Could you check a few things on this model? Use its own coordinates, in mm. A direction names the side the tool comes from. Give positions to 0.01 mm unless a question says otherwise; leave off trailing zeros. Order: outer loops, then holes, each group sorted by start corner. A loop starts at its lowest first (then second) coordinate and runs counter-clockwise, first axis right, second up. Notation, with made-up numbers: (29.25, -32) -> (34.25, -32) arc R10 ccw to (34.25, -21) -> close; hole circle Ø3 at (83.5, 9.5). An arc over 180 degrees is marked (long way). Answer as CSV lines item,"result". Start each with the question number.
(1) I need wall thicknesses on L1, parallel to X at y = 8.75, z = -36; L2, parallel to Z at x = -69, y = 4.5; L3, parallel to X at y = 8, z = 90.5. Which ranges of each line are inside material? Lowest first, please.
(2) I want a section at A-A (z = 49.5). Please give me the cut outline in (x, y).
(3) Will this pin go through, and if not, where does the flat tip stop? pin 1 Ø1 at (x, y) = (3.5, 7.5) entering from +Z.
(4) I want a section at B-B (y = 6.75). Give the number of separate pieces and of enclosed holes in the cut face, plus the area to 3 significant figures.
(5) On a 3-axis mill with a long thin cutter (end or side, diameter ignored), from which of +Z, -Z, +X, -X, +Y, -Y can I reach the whole of each face in a straight line? I mean faces 4 (the face through (-21.359, 6.056, -8.797)), 5 (the face through (-25.047, 6, 89)). Say none if no direction works.
(6) We'd pull the mould along Z, two halves only. Please class faces 1 (the face through (1, 1.6, 100)), 2 (the face through (1, 0, -1)), 3 (the face through (32, 6, 55.357)): released by +Z, released by -Z, zero draft, split by the parting line, or undercut.
```python
from build123d import *

# Parameters (mm, degrees)
EXTRUDE_1_DEPTH     = 10
CUT_EXTRUDE_1_DEPTH = 8
SKETCH_3_R          = 1.5875
CUT_EXTRUDE_2_DEPTH = 126.39936204


with BuildPart() as part:
    # Эскиз1 → Бобышка-Вытянуть1 (new body)
    with BuildSketch(Plane(origin=(0, 0, 0), x_dir=(1, 0, 0), z_dir=(0, 1, 0))):
        with BuildLine():
            Line((-72, 100), (72, 100))
            ThreePointArc((72, 100), (74.121320344, 99.121320344), (75, 97))
            Line((75, 97), (75, -97))
            ThreePointArc((75, -97), (74.121320344, -99.121320344), (72, -100))
            Line((72, -100), (-72, -100))
            ThreePointArc((-72, -100), (-74.121320344, -99.121320344), (-75, -97))
            Line((-75, -97), (-75, 97))
            ThreePointArc((-75, 97), (-74.121320344, 99.121320344), (-72, 100))
        make_face()
    extrude(amount=EXTRUDE_1_DEPTH)

    # Эскиз2 → Вырез-Вытянуть1 (cut)
    with BuildSketch(Plane(origin=(0, 10, 0), x_dir=(1, 0, 0), z_dir=(0, 1, 0))):
        with BuildLine():
            Line((22.5, 6), (22.5, -3.982244962))
            ThreePointArc((22.5, -3.982244962), (22.659034481, -4.946047285), (23.119276612, -5.807664407))
            Line((23.119276612, -5.807664407), (29.380723388, -13.973882215))
            ThreePointArc((29.380723388, -13.973882215), (29.840965519, -14.835499337), (30, -15.799301661))
            Line((30, -15.799301661), (30, -41.994552887))
            ThreePointArc((30, -41.994552887), (29.121320344, -44.115873231), (27, -44.994552887))
            Line((27, -44.994552887), (-27, -44.994552887))
            ThreePointArc((-27, -44.994552887), (-29.121320344, -44.115873231), (-30, -41.994552887))
            Line((-30, -41.994552887), (-30, -15.799301661))
            ThreePointArc((-30, -15.799301661), (-29.840965519, -14.835499337), (-29.380723388, -13.973882215))
            Line((-29.380723388, -13.973882215), (-23.119276612, -5.807664407))
            ThreePointArc((-23.119276612, -5.807664407), (-22.659034481, -4.946047285), (-22.5, -3.982244962))
            Line((-22.5, -3.982244962), (-22.5, 6))
            ThreePointArc((-22.5, 6), (-21.328427125, 8.828427125), (-18.5, 10))
            Line((-18.5, 10), (-7, 10))
            ThreePointArc((-7, 10), (-3.585786438, 8.585786438), (-5, 12))
            Line((-5, 12), (-5, 68))
            ThreePointArc((-5, 68), (-3.585786438, 71.414213562), (-7, 70))
            Line((-7, 70), (-63, 70))
            ThreePointArc((-63, 70), (-66.414213562, 71.414213562), (-65, 68))
            Line((-65, 68), (-65, 12))
            ThreePointArc((-65, 12), (-66.414213562, 8.585786438), (-63, 10))
            Line((-63, 10), (-51.5, 10))
            ThreePointArc((-51.5, 10), (-48.671572875, 8.828427125), (-47.5, 6))
            Line((-47.5, 6), (-47.5, -3.982244962))
            ThreePointArc((-47.5, -3.982244962), (-47.340965519, -4.946047285), (-46.880723388, -5.807664407))
            Line((-46.880723388, -5.807664407), (-40.619276612, -13.973882215))
            ThreePointArc((-40.619276612, -13.973882215), (-40.159034481, -14.835499337), (-40, -15.799301661))
            Line((-40, -15.799301661), (-40, -52.357484611))
            ThreePointArc((-40, -52.357484611), (-39.121320344, -54.478804954), (-37, -55.357484611))
            Line((-37, -55.357484611), (-28.046989376, -55.357484611))
            ThreePointArc((-28.046989376, -55.357484611), (-25.925669032, -56.236164267), (-25.046989376, -58.357484611))
            Line((-25.046989376, -58.357484611), (-25.046989376, -58.607484611))
            ThreePointArc((-25.046989376, -58.607484611), (-25.925669032, -60.728804954), (-28.046989376, -61.607484611))
            Line((-28.046989376, -61.607484611), (-31.247779241, -61.607484611))
            ThreePointArc((-31.247779241, -61.607484611), (-32.020054596, -61.70858986), (-32.74027589, -62.00509076))
            Line((-32.74027589, -62.00509076), (-37.020569868, -64.459878461))
            ThreePointArc((-37.020569868, -64.459878461), (-37.740791162, -64.756379361), (-38.513066517, -64.857484611))
            Line((-38.513066517, -64.857484611), (-47.380723388, -64.857484611))
            ThreePointArc((-47.380723388, -64.857484611), (-49.502043731, -65.736164267), (-50.380723388, -67.857484611))
            Line((-50.380723388, -67.857484611), (-50.380723388, -100))
            Line((-50.380723388, -100), (-43.380723388, -100))
            Line((-43.380723388, -100), (-43.380723388, -74.857484611))
            ThreePointArc((-43.380723388, -74.857484611), (-42.502043731, -72.736164267), (-40.380723388, -71.857484611))
            Line((-40.380723388, -71.857484611), (-38.513066517, -71.857484611))
            ThreePointArc((-38.513066517, -71.857484611), (-37.740791162, -71.95858986), (-37.020569868, -72.25509076))
            Line((-37.020569868, -72.25509076), (-32.74027589, -74.709878461))
            ThreePointArc((-32.74027589, -74.709878461), (-32.020054596, -75.006379361), (-31.247779241, -75.107484611))
            Line((-31.247779241, -75.107484611), (-28.046989376, -75.107484611))
            ThreePointArc((-28.046989376, -75.107484611), (-25.925669032, -75.986164267), (-25.046989376, -78.107484611))
            Line((-25.046989376, -78.107484611), (-25.046989376, -100))
            Line((-25.046989376, -100), (25.046989376, -100))
            Line((25.046989376, -100), (25.046989376, -78.107484611))
            Line((25.046989376, -78.107484611), (25.046989376, -58.357484611))
            ThreePointArc((25.046989376, -58.357484611), (25.925669032, -56.236164267), (28.046989376, -55.357484611))
            Line((28.046989376, -55.357484611), (37, -55.357484611))
            ThreePointArc((37, -55.357484611), (39.121320344, -54.478804954), (40, -52.357484611))
            Line((40, -52.357484611), (40, -15.799301661))
            ThreePointArc((40, -15.799301661), (40.159034481, -14.835499337), (40.619276612, -13.973882215))
            Line((40.619276612, -13.973882215), (46.880723388, -5.807664407))
            ThreePointArc((46.880723388, -5.807664407), (47.340965519, -4.946047285), (47.5, -3.982244962))
            Line((47.5, -3.982244962), (47.5, 6))
            ThreePointArc((47.5, 6), (48.671572875, 8.828427125), (51.5, 10))
            Line((51.5, 10), (63, 10))
            ThreePointArc((63, 10), (66.414213562, 8.585786438), (65, 12))
            Line((65, 12), (65, 68))
            ThreePointArc((65, 68), (66.414213562, 71.414213562), (63, 70))
            Line((63, 70), (7, 70))
            ThreePointArc((7, 70), (3.585786438, 71.414213562), (5, 68))
            Line((5, 68), (5, 12))
            ThreePointArc((5, 12), (3.585786438, 8.585786438), (7, 10))
            Line((7, 10), (18.5, 10))
            ThreePointArc((18.5, 10), (21.328427125, 8.828427125), (22.5, 6))
        make_face()
    extrude(amount=-CUT_EXTRUDE_1_DEPTH, mode=Mode.SUBTRACT)

    # Эскиз3 → Вырез-Вытянуть2 (cut, through all)
    with BuildSketch(Plane(origin=(0, 10, 0), x_dir=(1, 0, 0), z_dir=(0, 1, 0))):
        with Locations(Location((-69, 94, 0), (0, 0, 270))):
            Circle(SKETCH_3_R)
        with Locations(Location((0, 94, 0), (0, 0, 270))):
            Circle(SKETCH_3_R)
        with Locations(Location((69, 94, 0), (0, 0, 270))):
            Circle(SKETCH_3_R)
        with Locations(Location((-69, -34, 0), (0, 0, 90))):
            Circle(SKETCH_3_R)
        with Locations(Location((69, -34, 0), (0, 0, 90))):
            Circle(SKETCH_3_R)
        with Locations(Location((0, -34, 0), (0, 0, 90))):
            Circle(SKETCH_3_R)
        with Locations(Location((69, -94, 0), (0, 0, 90))):
            Circle(SKETCH_3_R)
        with Locations(Location((-69, -94, 0), (0, 0, 90))):
            Circle(SKETCH_3_R)
        with Locations(Location((0, 34, 0), (0, 0, 270))):
            Circle(SKETCH_3_R)
        with Locations(Location((69, 34, 0), (0, 0, 270))):
            Circle(SKETCH_3_R)
        with Locations(Location((-69, 34, 0), (0, 0, 270))):
            Circle(SKETCH_3_R)
    extrude(amount=-CUT_EXTRUDE_2_DEPTH, mode=Mode.SUBTRACT)


solid = part.part
```
Final values:
1,L1,"-75 to -65, -5 to 5, 65 to 75"
1,L2,"-100 to -95.59, -92.41 to -35.59, -32.41 to 32.41, 35.59 to 92.41, 95.59 to 100"
1,L3,"-75 to -50.38, -43.38 to -25.05, 25.05 to 75"
2,outline,"(-75, 0) -> (75, 0) -> (75, 10) -> (40, 10) -> (40, 2) -> (-40, 2) -> (-40, 10) -> (-75, 10) -> close"
3,pin 1,"z = 44.99"
4,separate pieces,"2"
4,enclosed holes,"11"
4,area,"17,400 mm²"
5,face 4,"+Y"
5,face 5,"+Z, +Y"
6,face 1,"released by +Z"
6,face 2,"zero draft"
6,face 3,"undercut"
